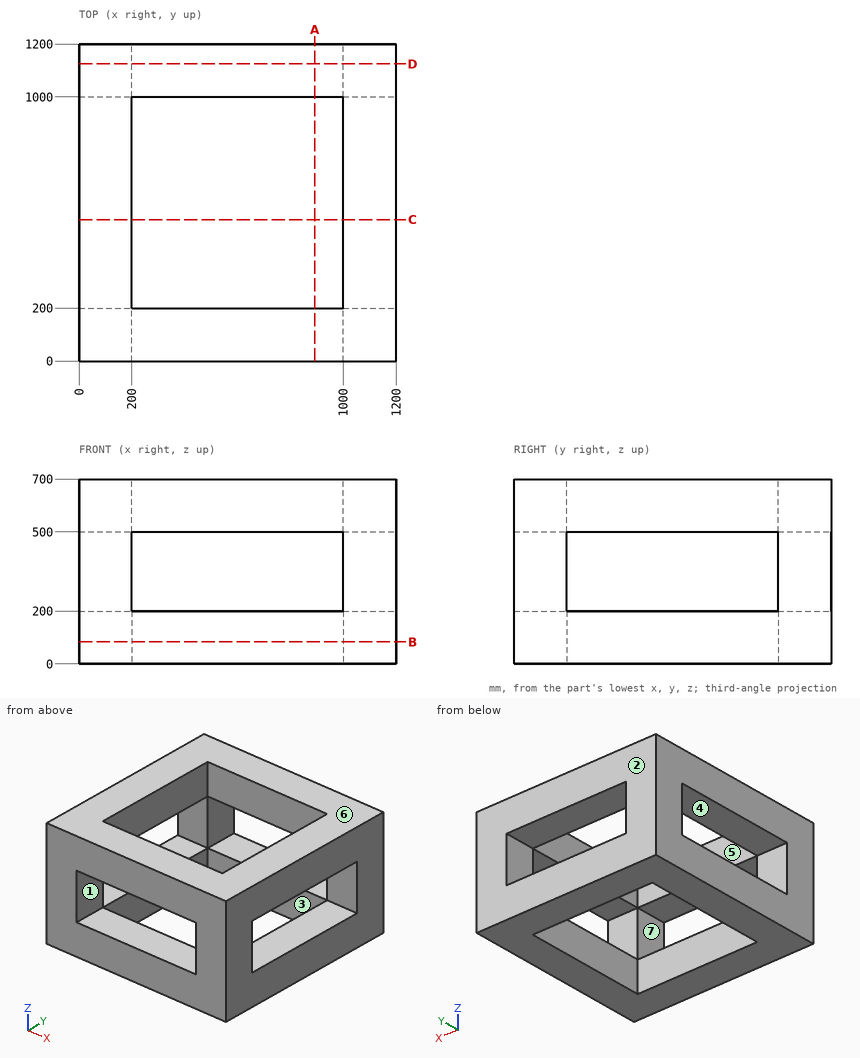
Input: dimensioned drawing with shaded views. Units: mm. Origin: part minimum x, y, z. A direction names the side the tool comes from. Give positions to 0.01 mm unless a question says otherwise; leave off trailing zeros. Write each loop counter-clockwise with the first axis right and the second up, starting at its lowest first coordinate (ties: lowest second). Pieces come first, ordered by that corner, then holes. Notation, with made-up numbers: (44, -31) -> (49, -31) arc R14 cw to (49, -20) -> close; hole circle Ø4 at (-26.5, 42). An arc over 180 degrees is marked (long way). Return JSON: item names as keys, results as strings. Group by question number.
1. Mould query, pull axis Y, two halves, no side actions, for the marked faces 1, 2 and 3. Classes: +Y half, -Y half, draft (parallel to the pull), parting line (faces both ways), or undercut.
2. Section B-B, the plane z = 83. Output: boundary loops of the cut face in (x, y), then the cut area to 3 significant figures.
3. Section D-D, the plane y = 1124.5. Output: boundary loops of the cut face in (x, z), then the cut area to 3 significant figures.
4. Section A-A, the plane x = 893. Output: boundary loops of the cut face in (y, z), then the cut area to 3 significant figures.
5. Material intervals for line 1 (Z direction, x = 1007, y = 363); line 2 (Y direction, x = 345, z = 532.5), sorted ascending. Write a range as from..to.
6. Access query for the marked faces 4, 5, 6 and 7. Directions: +Z, -Z, +X, -X, +Y, -Y. A direction counts if a zero-diameter tool reaches every point of the face in a straight line with its end or side. Return the directions, or none.
Determined:
{
 "1": {"face 1": "draft", "face 2": "+Y half", "face 3": "undercut"},
 "2": {"outline": "(0, 0) -> (1200, 0) -> (1200, 1200) -> (0, 1200) -> close; hole (200, 200) -> (1000, 200) -> (1000, 1000) -> (200, 1000) -> close", "area": "800,000 mm2"},
 "3": {"outline": "(0, 0) -> (1200, 0) -> (1200, 700) -> (0, 700) -> close; hole (200, 200) -> (1000, 200) -> (1000, 500) -> (200, 500) -> close", "area": "600,000 mm2"},
 "4": {"outline": "(0, 0) -> (200, 0) -> (200, 200) -> (0, 200) -> close; (0, 500) -> (200, 500) -> (200, 700) -> (0, 700) -> close; (1000, 0) -> (1200, 0) -> (1200, 200) -> (1000, 200) -> close; (1000, 500) -> (1200, 500) -> (1200, 700) -> (1000, 700) -> close", "area": "160,000 mm2"},
 "5": {"line 1": "z = 0..200, 500..700", "line 2": "y = 0..200, 1000..1200"},
 "6": {"face 4": "+X, -X", "face 5": "+Z, -Z", "face 6": "+Z, +X, -X, +Y, -Y", "face 7": "+Y, -Y"}
}
